Answer from the drawing. Dimensions are ordinates in mm from the lowest x, y and z of the part. A direction names the side the tool comes from. Give positions to 0.01 mm unless a question says otherwise; leave off trailing zeros. Loops run counter-clockwise (first coordinate to the right, second up) from the corner with the lowest first, then second, coordinate; pieces in that order, holes last. Notation, with made-up numbers: (44, 9.25) -> (88, 9.25) arc R11 cw to (88, 27.25) -> close; hole circle Ø11 at (15.5, 37). An arc over 180 degrees is marked (long way). Return JSON: item names as keys, results as strings. Group by question number.
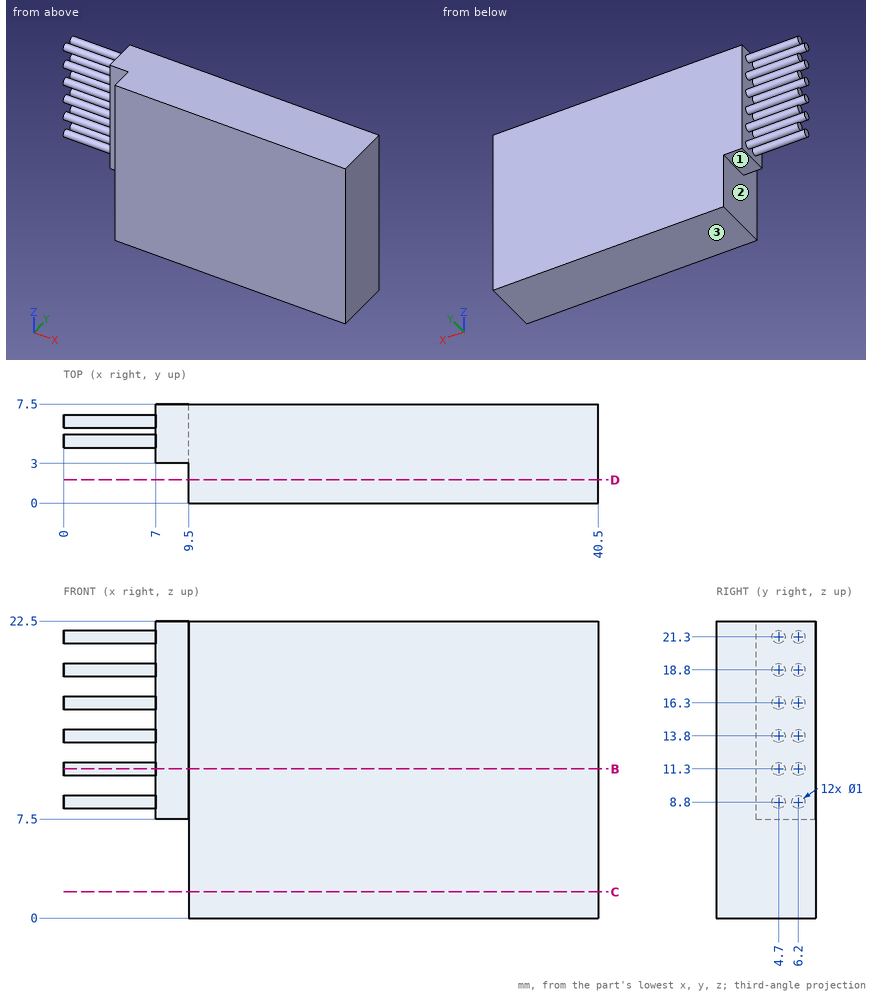
1. Which of the six approach directions +Z, -Z, +X, -X, +Y, -Y give full straight-line access (tool end or side, diameter ignored) to the marked faces 1, 2 and 3?
2. Flat-ended cylindrical pins translate along their axes: pin 1 Ø2 at (x, z) = (8, 18) entering from -Y; pin 2 Ø1.2 at (x, y) = (8.5, 6) entering from -Z; pin 3 Ø2 at (y, z) = (1, 18.5) entering from -X. Find the tip coordinate at first contact, or state that the pin passes through.
3. Straight lines are drawn through the part: line 1 (X direction, y = 1.5, z = 20.5); line 2 (Z direction, x = 8, y = 4); line 3 (X direction, y = 4.5, z = 17.75). For each, find the intervals that lie inside material, in ascending order. Write a range as from..to.
4. Section D-D on y = 1.75 is taken. Determine the outline of the cut face in (x, z).
5. Section B-B on z = 11.3 is taken. Determine the outline of the cut face in (x, y).
6. Section C-C on z = 2 is taken. Determine the outline of the cut face in (x, y).
Completed:
{
 "1": {"face 1": "-Z, -X, +Y, -Y", "face 2": "-Z, -X, -Y", "face 3": "-Z, +X, -X, +Y, -Y"},
 "2": {"pin 1": "stops at y = 3", "pin 2": "stops at z = 7.5", "pin 3": "stops at x = 9.5"},
 "3": {"line 1": "x = 9.5..40.5", "line 2": "z = 7.5..22.5", "line 3": "x = 7..40.5"},
 "4": {"outline": "(9.5, 0) -> (40.5, 0) -> (40.5, 22.5) -> (9.5, 22.5) -> close"},
 "5": {"outline": "(0, 4.2) -> (7, 4.2) -> (7, 3) -> (9.5, 3) -> (9.5, 0) -> (40.5, 0) -> (40.5, 7.5) -> (7, 7.5) -> (7, 6.7) -> (0, 6.7) -> (0, 5.7) -> (7, 5.7) -> (7, 5.2) -> (0, 5.2) -> close"},
 "6": {"outline": "(9.5, 0) -> (40.5, 0) -> (40.5, 7.5) -> (9.5, 7.5) -> close"}
}
